Could you check a few things on this model? Use its own coordinates, in mm. Round coordinates to 2 decimals unless told otherwise and drop trailing zeros. Write each loop counter-clockwise with the first axis right and the second up, starting at its lowest first coordinate (ties: lowest second). Pieces come first, ordered by that corner, then holes. Notation, with made-up numbers: (-16.75, 14.5) - (-10.75, 14.5) arc R26 ccw to (-10.75, 35.5) - close; hole circle Ø9 at (-28, 8.25). An arc over 180 degrees is marked (long way). Put each result on its own line as item: value.
from build123d import *

# Parameters (mm, degrees)
BOSS_EXTRUDE1_DEPTH = 1.5875


with BuildPart() as part:
    # Sketch2 → Boss-Extrude1 (new, symmetric)
    with BuildSketch(Plane.XY):
        with BuildLine():
            ThreePointArc((-120.098895727, 19.05), (0.406748907, 139.2017743), (120.203613722, 18.343301545))
            ThreePointArc((120.203613722, 18.343301545), (101.067699546, -47.629728931), (50.138751442, -93.726))
            ThreePointArc((50.138751442, -93.726), (0.040174098, -101.514794876), (-50.058403246, -93.726))
            ThreePointArc((-50.058403246, -93.726), (-101.163912713, -47.327889321), (-120.098895727, 19.05))
        make_face()
        with BuildLine():
            ThreePointArc((-104.858895727, 19.05), (0.361930242, 123.961840203), (104.963877332, 18.432938489))
            ThreePointArc((104.963877332, 18.432938489), (88.446745877, -39.065849025), (44.40486057, -79.553359885))
            ThreePointArc((44.40486057, -79.553359885), (0.040463589, -86.274794876), (-44.323959374, -79.553531384))
            ThreePointArc((-44.323959374, -79.553531384), (-88.517658334, -38.801393502), (-104.858895727, 19.05))
        make_face(mode=Mode.SUBTRACT)
    extrude(amount=BOSS_EXTRUDE1_DEPTH, both=True)


solid = part.part
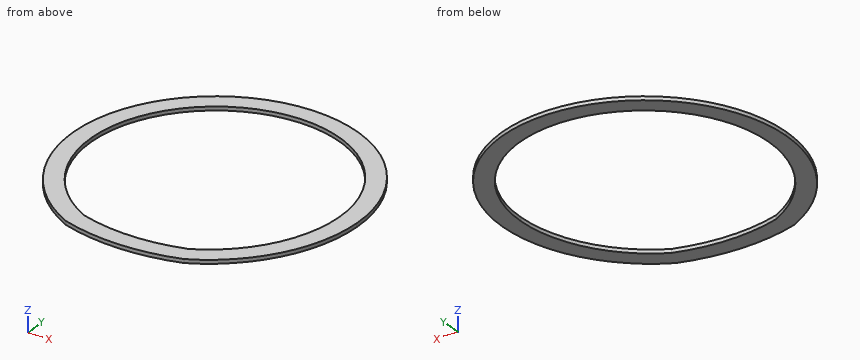
(1) Imagine slicing it at B-B, the plane y = 25. List the corners of the cut face in (x, z) for me.
Values found:
outline: (-119.95, -1.59) - (-104.69, -1.59) - (-104.69, 1.59) - (-119.95, 1.59) - close; (104.8, -1.59) - (120.06, -1.59) - (120.06, 1.59) - (104.8, 1.59) - close
(2) Please list where these lines run through material, in increasing order: probe 1 along X at (y, z) = (34, -1.3); probe 2 along Y at (x, z) = (-8.5, 0.75); probe 3 along Y at (x, z) = (30.5, 1.3). Write a range as from..to.
Values found:
probe 1: x = -119.17..-103.79, 103.9..119.27
probe 2: y = -101.29..-86.03, 123.61..138.9
probe 3: y = -98.68..-83.14, 119.45..135.28
(3) I'm going to push flat-ended pins straight in: pin 1 (1.5 mm diameter, centred on x = 33.5, z = -1, fed in from +Y); pin 2 (1.5 mm diameter, centred on x = -57.5, z = 1, fed in from -Y); pin 3 (8 mm diameter, centred on x = 87, y = -66.5, fed in from -Z); pin 4 (1.5 mm diameter, centred on y = -77, z = -0.5, fed in from -X). Where does each tip first touch, or does it pass through?
Values found:
pin 1: stops at y = 134.67
pin 2: stops at y = -90.16
pin 3: stops at z = -1.59
pin 4: stops at x = -76.43
(4) Imagine slicing it at A-A, the plane z = -0.45. List the corners of the cut face in (x, y) for me.
Values found:
outline: (-120.1, 19.05) arc R125.81 ccw to (-50.06, -93.73) arc R165.01 ccw to (50.14, -93.73) arc R125.85 ccw to (120.2, 18.34) arc R120.15 ccw (long way) to start; hole (-104.86, 19.05) arc R110.57 ccw to (-44.32, -79.55) arc R149.77 ccw to (44.4, -79.55) arc R110.61 ccw to (104.96, 18.43) arc R104.91 ccw (long way) to start
(5) Imagine slicing it at C-C, the plane x = -22. List the corners of the cut face in (y, z) for me.
Values found:
outline: (-100.04, -1.59) - (-84.64, -1.59) - (-84.64, 1.59) - (-100.04, 1.59) - close; (121.62, -1.59) - (137.16, -1.59) - (137.16, 1.59) - (121.62, 1.59) - close
